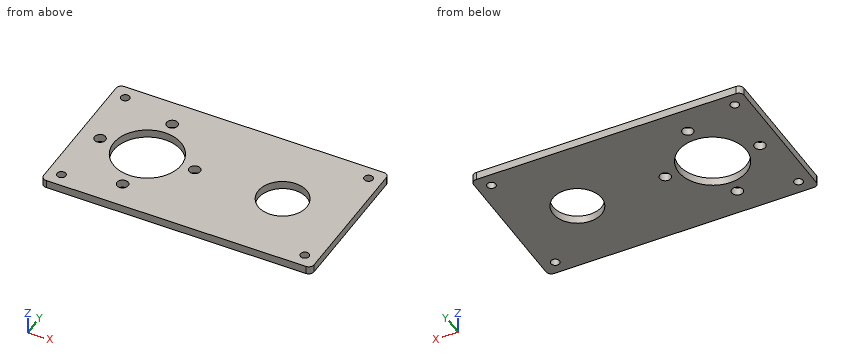
Autodesk Inventor part; units mm, degrees
ref_plane "YZ Plane" through (0, 0, 0) normal (1, 0, 0) x (0, 1, 0)
ref_plane "XZ Plane" through (0, 0, 0) normal (0, 1, 0) x (-1, 0, 0)
ref_plane "XY Plane" through (0, 0, 0) normal (0, 0, 1) x (1, 0, 0)
sketch "スケッチ1" plane through (0, 0, 0) normal (0, 0, 1) x (1, 0, 0)
  line L0 (50, -27.5) -> (-50, -27.5)
  line L1 (-50, -27.5) -> (-50, 27.5)
  line L2 (-50, 27.5) -> (50, 27.5)
  line L3 (50, 27.5) -> (50, -27.5)
  line L4 (50, -27.5) -> (-50, 27.5) construction
  line L5 (-50, -27.5) -> (50, 27.5) construction
  circle A0 centre (0, 0) radius 25
  line L6 (-50, 0) -> (50, 0)
  circle A1 centre (25, 0) radius 9
  circle A2 centre (-25, 0) radius 12.5
  circle A3 centre (-25, 0) radius 17.5
  circle A4 centre (-25, 17.5) radius 2.05
  circle A5 centre (-42.5, 0) radius 2.05
  circle A6 centre (-25, -17.5) radius 2.05
  circle A7 centre (-7.5, 0) radius 2.05
  dimension "d5" = 35
  dimension "d0" = 100
  dimension "d1" = 55
  dimension "d2" = 50
  dimension "d3" = 18
  dimension "d4" = 25
  dimension "d6" = 4.1
  dimension "d9" = 360
  dimension "d11" = 25
extrude "押し出し1" add sketch "スケッチ1" along normal blind 3 contours L0 L1 L6 A5 A3 A6 A0 A1 L3 | L6 A1 A0 A3 A4 A5 L1 L2 L3 | A1 L6 A7 A3 A0 | A0 A3 A7 L6 A1 | A3 A4 A0 A2 L6 A5 | A5 L6 A2 A0 A3 A6 | A3 A7 L6 A2 A0 | A0 A2 L6 A7 A3
sketch "スケッチ2" plane through (0, 0, 3) normal (0, 0, 1) x (1, 0, 0)
  line L0 (50, 27.5) -> (-50, 27.5)
  line L1 (-50, 27.5) -> (-50, -27.5)
  line L2 (-50, -27.5) -> (50, -27.5)
  line L3 (50, -27.5) -> (50, 27.5)
  circle A0 centre (25, 0) radius 9
  circle A1 centre (-7.5, 0) radius 2.05
  circle A2 centre (-25, 17.5) radius 2.05
  circle A3 centre (-42.5, 0) radius 2.05
  circle A4 centre (-25, -17.5) radius 2.05
  circle A5 centre (-25, 0) radius 12.5
  line L4 (-45, 22.5) -> (45, 22.5)
  line L5 (45, 22.5) -> (45, -22.5)
  line L6 (45, -22.5) -> (-45, -22.5)
  line L7 (-45, -22.5) -> (-45, 22.5)
  point P0 (0, 0)
  dimension "d14" = 5
hole "穴1" at (-45, 22.5, 3) at (-45, -22.5, 3) at (45, -22.5, 3) at (45, 22.5, 3) direction (0, 0, -1) diameter 3.2 end through all
fillet "フィレット1" radius 2 4 edges at (-50, 27.5, 1.5) (50, 27.5, 1.5) (50, -27.5, 1.5) (-50, -27.5, 1.5)
sketch "スケッチ3" plane through (0, 0, 3) normal (0, 0, 1) x (1, 0, 0)
  arc A0 (-50, -25.5) -> (-48, -27.5) centre (-48, -25.5) ccw
  line L0 (-48, -27.5) -> (48, -27.5)
  arc A1 (48, -27.5) -> (50, -25.5) centre (48, -25.5) ccw
  line L1 (50, -25.5) -> (50, 25.5)
  arc A2 (50, 25.5) -> (48, 27.5) centre (48, 25.5) ccw
  line L2 (48, 27.5) -> (-48, 27.5)
  arc A3 (-48, 27.5) -> (-50, 25.5) centre (-48, 25.5) ccw
  line L3 (-50, 25.5) -> (-50, -25.5)
  circle A4 centre (45, 22.5) radius 1.6
  circle A5 centre (45, -22.5) radius 1.6
  circle A6 centre (-45, -22.5) radius 1.6
  circle A7 centre (-45, 22.5) radius 1.6
  circle A8 centre (25, 0) radius 9
  circle A9 centre (-7.5, 0) radius 2.05
  circle A10 centre (-25, 17.5) radius 2.05
  circle A11 centre (-42.5, 0) radius 2.05
  circle A12 centre (-25, -17.5) radius 2.05
  circle A13 centre (-25, 0) radius 12.5
  point P0 (0, 0)
equation "\"d11\" = -0.5 * d2 + 0.5 * d0"
properties part number "xx_plate_motor"
Verification items for the finished model (mm, model axes). Give positions to 0.01 mm unless a question says otherwise; leave off trailing zeros. Write each loop counter-clockwise with the first axis right and the second up, starting at its lowest first coordinate (ties: lowest second). Pieces come first, ordered by that corner, then holes. Notation, with made-up numbers: M 44,16.5 L 59,16.5 A18 ccw 59,38.5 Z; hole C -23.5,30.25 d9. An arc over 180 degrees is marked long. Use CSV: the item, a comma, the result in double quotes.
1) Cross-section at A-A (y = 17.5). Enter the section's corners in (x, z).
Final values:
outline,"M -50,0 L -27.05,0 L -27.05,3 L -50,3 Z; M -22.95,0 L 50,0 L 50,3 L -22.95,3 Z"
2) Cross-section at C-C (z = 2.4). State how many separate pieces and enclosed holes the cut face has, plus the area to 3 significant figures.
Final values:
separate pieces,"1"
enclosed holes,"10"
area,"4,670 mm²"
3) Cross-section at B-B (x = 25). Enter the section's corners in (y, z), plus the area to 3 significant figures.
Final values:
outline,"M -27.5,0 L -9,0 L -9,3 L -27.5,3 Z; M 9,0 L 27.5,0 L 27.5,3 L 9,3 Z"
area,"111 mm²"
4) Material ranges on line 1 along X through (y, z) = (22.5, 2.3); line 2 along Y through (x, z) = (-45, 1.2); line 3 along X through (y, z) = (1.5, 2.5), recorded low to high.
Final values:
line 1,"-50 to -46.6, -43.4 to 43.4, 46.6 to 50"
line 2,"-27.5 to -24.1, -20.9 to 20.9, 24.1 to 27.5"
line 3,"-50 to -43.9, -41.1 to -37.41, -12.59 to -8.9, -6.1 to 16.13, 33.87 to 50"
